For this review, use the dimensioned drawing (mm, ordinates from the lowest corner) and the shaded views. Round coordinates to 2 decimals unless told otherwise and drop trailing zeros. Write each loop counter-clockwise with the first axis right and the second up, starting at its lowest first coordinate (ties: lowest second). Pieces come first, ordered by that corner, then holes. Notation, with made-up numbers: (10.5, 54.5) -> (31.5, 54.5) arc R7 cw to (31.5, 58.5) -> close; hole circle Ø6 at (-30, -18). An arc over 180 degrees is marked (long way). Answer as CSV lines item,"result". Start each with the question number.
Item 1: Take a section at B-B on y = 7. Give the boundary of the cut face in (x, z) (1 decimal), then the cut area to 3 significant figures.
Item 2: For pin 1 Ø6 at (y, z) = (7, 32) entering from +X; pin 2 Ø5.5 at (x, y) = (94, 8.5) entering from +Z (1 decimal); pin 3 Ø5 at (y, z) = (3, 33) entering from -X (1 decimal); pin 4 Ø5.5 at (x, y) = (6, 7) entering from -Z, all flat-tipped, find the tip position at first contact; note any pin that passes through.
Item 3: Take a section at A-A on z = 36.5. Give the boundary of the cut face in (x, y) (1 decimal).
Item 4: Take a section at D-D on x = 94. Give the boundary of the cut face in (y, z) (1 decimal).
Item 5: Mouldability with a two-part tool opening along X and no side actions: class the marked faces 1, 2 and 3 as +X half, -X half, draft (parallel to the pull), parting line (faces both ways), or undercut.
Item 6: Wall thickness on probe 1 along Y at (x, z) = (94, 4); probe 2 along Z at (x, y) = (51, 7); probe 3 along X at (y, z) = (8.25, 11) (1 decimal): over which ranges is each line inside the solid? List them lowest first. Write a range as from..to.
Item 7: Take a section at C-C on y = 2.5. Give the boundary of the cut face in (x, z) (1 decimal).
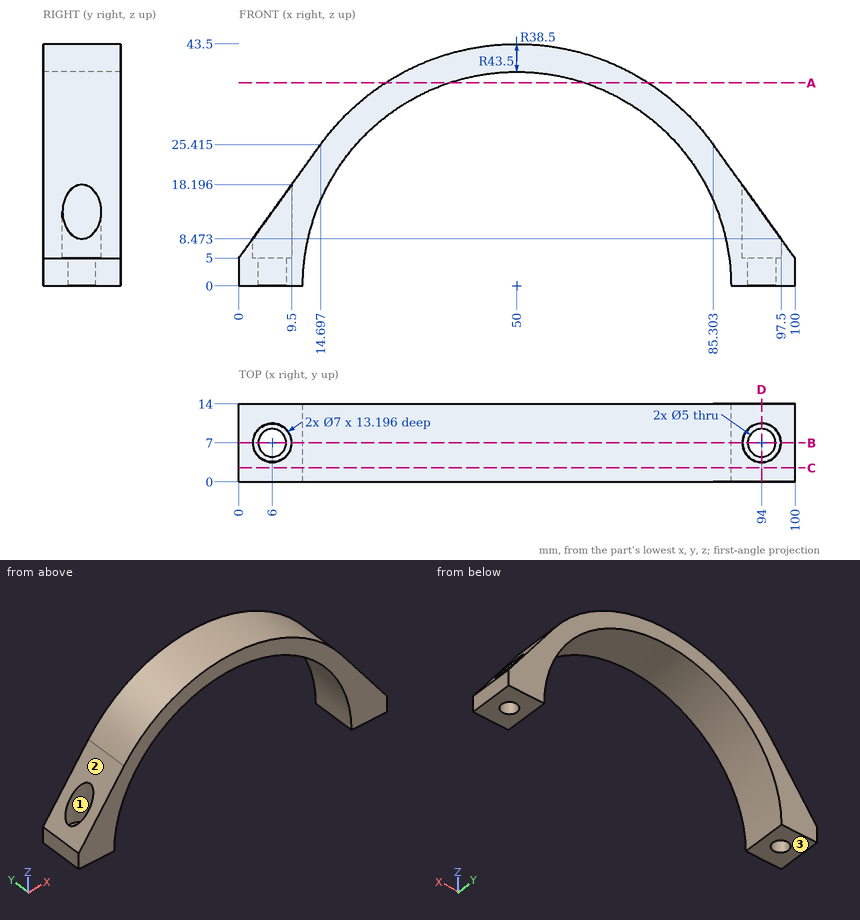
Output values:
1,outline,"(0, 0) -> (3.5, 0) -> (3.5, 5) -> (2.5, 5) -> (2.5, 8.5) -> (0, 5) -> close; (8.5, 0) -> (11.5, 0) arc R38.5 cw to (88.5, 0) -> (91.5, 0) -> (91.5, 5) -> (90.5, 5) -> (90.5, 18.2) -> (85.3, 25.4) arc R43.5 ccw to (14.7, 25.4) -> (9.5, 18.2) -> (9.5, 5) -> (8.5, 5) -> close; (96.5, 0) -> (100, 0) -> (100, 5) -> (97.5, 8.5) -> (97.5, 5) -> (96.5, 5) -> close"
1,area,"641 mm^2"
2,pin 1,"stops at x = 82.42"
2,pin 2,"stops at z = 17"
2,pin 3,"stops at x = 19"
2,pin 4,"stops at z = 0"
3,outline,"(26.3, 0) -> (37.8, 0) -> (37.8, 14) -> (26.3, 14) -> close; (62.2, 0) -> (73.7, 0) -> (73.7, 14) -> (62.2, 14) -> close"
4,outline,"(0, 0) -> (4.5, 0) -> (4.5, 5) -> (3.5, 5) -> (3.5, 13.3) -> (0, 13.3) -> close; (9.5, 0) -> (14, 0) -> (14, 13.3) -> (10.5, 13.3) -> (10.5, 5) -> (9.5, 5) -> close"
5,face 1,"undercut"
5,face 2,"-X half"
5,face 3,"draft"
6,probe 1,"y = 0..4.5, 9.5..14"
6,probe 2,"z = 38.49..43.49"
6,probe 3,"x = 9.3..13.1, 86.9..90.7"
7,outline,"(0, 0) -> (11.5, 0) arc R38.5 cw to (88.5, 0) -> (100, 0) -> (100, 5) -> (85.3, 25.4) arc R43.5 ccw to (14.7, 25.4) -> (0, 5) -> close"
